```python
from build123d import *

# Parameters (mm, degrees)
SKETCH_1_W          = 50
SKETCH_1_H          = 62
EXTRUDE_1_DEPTH     = 24
FILLET_1_R          = 25
SKETCH_2_R          = 15
CUT_EXTRUDE_1_DEPTH = 30
SKETCH_3_R          = 17.5
CUT_EXTRUDE_2_DEPTH = 3


with BuildPart() as part:
    # 草图1 → 拉伸1 (new body)
    with BuildSketch(Plane.XY):
        with Locations((25, -31)):
            Rectangle(SKETCH_1_W, SKETCH_1_H)
    extrude(amount=EXTRUDE_1_DEPTH)

    # 圆角1
    fillet_1_edges = [part.edges().sort_by_distance(p)[0] for p in [
        (0, -62, 12),
        (50, -62, 12),
    ]]
    fillet(fillet_1_edges, radius=FILLET_1_R - 0.0001)  # a hair under: the kernel refuses the full size

    # 草图2 → 切除-拉伸1 (cut)
    with BuildSketch(Plane(origin=(0, 0, 0), x_dir=(-1, 0, 0), z_dir=(0, 0, -1))):
        with Locations((-25, -37)):
            Circle(SKETCH_2_R)
    extrude(amount=-CUT_EXTRUDE_1_DEPTH, mode=Mode.SUBTRACT)

    # 草图3 → 切除-拉伸2 (cut)
    with BuildSketch(Plane.XY.offset(24)):
        with Locations((25, -37)):
            Circle(SKETCH_3_R)
    extrude(amount=-CUT_EXTRUDE_2_DEPTH, mode=Mode.SUBTRACT)


solid = part.part
```
Here's how the part is built. I have some questions about the finished solid (model axes, mm). A direction names the side the tool comes from. Round coordinates to 2 decimals unless told otherwise and drop trailing zeros. Write each loop counter-clockwise with the first axis right and the second up, starting at its lowest first coordinate (ties: lowest second). Pieces come first, ordered by that corner, then holes.
Q1. If we section it at C-C on x = 15: Write out the boundary of the cut face in (y, z), plus the area to 3 significant figures.
Q2. Which directions (+Z, -Z, +X, -X, +Y, -Y) give clear straight access to the entire face, cutting with the end or side of a thin tool? Please do faces 5 (the flat face through (50, -19, 12)), 6 (the cylindrical face through (12.102, -25.173, 22.521)).
Q3. If we section it at B-B on y = -50: Write out the boundary of the cut face in (x, z), plus the area to 3 significant figures.
Q4. If we section it at D-D on x = 41: Write out the boundary of the cut face in (y, z).
Q5. If we mould it in two halves opening along X, with no side actions, what happens to faces 1 (the cylindrical face through (36.056, -26.862, 10.353)), 2 (the flat face through (38, -29, 21)), 3 (the flat face through (0, -19, 12)), 4 (the flat face through (25, 0, 12))? For each: +X half, -X half, draft (parallel to the pull), parting line (faces both ways), or undercut.
Q6. Will these pins go through, and if not, where does the flat tip stop? P1, Ø17.5, axis at x = 17.5, y = -36.5, coming from the +Z side; P2, Ø12, axis at x = 28, z = 8, coming from the +Y side; P3, Ø1.5, axis at y = -39.5, z = 9, coming from the -X side.
Q7. Please list where these lines run through material, in increasing order: probe 1 along Y at (x, z) = (25, 22.7); probe 2 along Y at (x, z) = (25, 13.5); probe 3 along X at (y, z) = (-50, 13.75).
Answer below:
1. outline: (-59.91, 0) - (-48.18, 0) - (-48.18, 21) - (-51.36, 21) - (-51.36, 24) - (-59.91, 24) - close; (-25.82, 0) - (0, 0) - (0, 24) - (-22.64, 24) - (-22.64, 21) - (-25.82, 21) - close
1. area: 882 mm2
2. face 5: +Z, -Z, +X, +Y, -Y
2. face 6: +Z
3. outline: (3.65, 0) - (17.52, 0) - (17.52, 21) - (13.28, 21) - (13.28, 24) - (3.65, 24) - close; (32.48, 0) - (46.35, 0) - (46.35, 24) - (36.72, 24) - (36.72, 21) - (32.48, 21) - close
3. area: 640 mm2
4. outline: (-56.21, 0) - (0, 0) - (0, 24) - (-29.91, 24) - (-29.91, 21) - (-44.09, 21) - (-44.09, 24) - (-56.21, 24) - close
5. face 1: undercut
5. face 2: undercut
5. face 3: -X half
5. face 4: draft
6. P1: stops at z = 21
6. P2: stops at y = 0
6. P3: stops at x = 0.06
7. probe 1: y = -62 to -54.5, -19.5 to 0
7. probe 2: y = -62 to -52, -22 to 0
7. probe 3: x = 3.65 to 17.52, 32.48 to 46.35
